```python
from build123d import *

# Parameters (mm, degrees)
BOSS_EXTRUDE1_START = -10
SKETCH2_R           = 20
BOSS_EXTRUDE1_DEPTH = 30
SKETCH5_R           = 20
SKETCH5_R_2         = 11
CUT_EXTRUDE1_DEPTH  = 10
SKETCH7_R           = 20
BOSS_EXTRUDE2_DEPTH = 50
CUT_EXTRUDE2_DEPTH  = 50
CUT_EXTRUDE3_START  = -7.5
CUT_EXTRUDE3_DEPTH  = 87.335902125
SKETCH10_R          = 7
CUT_EXTRUDE4_DEPTH  = 77.23263398


with BuildPart() as part:
    # Sketch2 → Boss-Extrude1 (new body)
    with BuildSketch(Plane.XY.offset(BOSS_EXTRUDE1_START)):
        Circle(SKETCH2_R)
    extrude(amount=BOSS_EXTRUDE1_DEPTH)

    # Sketch5 → Cut-Extrude1 (cut)
    with BuildSketch(Plane(origin=(0, 0, -10), x_dir=(-1, 0, 0), z_dir=(0, 0, -1))):
        Circle(SKETCH5_R)
        Circle(SKETCH5_R_2, mode=Mode.SUBTRACT)
    extrude(amount=-CUT_EXTRUDE1_DEPTH, mode=Mode.SUBTRACT)

    # Sketch7 → Boss-Extrude2 (add)
    with BuildSketch(Plane.XY.offset(20)):
        with Locations(Location((0, 0, 0), (0, 0, 180))):
            Circle(SKETCH7_R)
    extrude(amount=BOSS_EXTRUDE2_DEPTH)

    # Sketch8 → Cut-Extrude2 (cut)
    with BuildSketch(Plane.XY.offset(70)):
        with BuildLine():
            ThreePointArc((15, 0), (13.608051098, 6.310383928), (9.690540625, 11.449603591))
            Line((9.690540625, 11.449603591), (10.389343078, -10.819498621))
            ThreePointArc((10.389343078, -10.819498621), (13.799277991, -5.880469957), (15, 0))
        make_face()
    extrude(amount=-CUT_EXTRUDE2_DEPTH, mode=Mode.SUBTRACT)

    # Sketch9 → Cut-Extrude3 (cut, through all)
    with BuildSketch(Plane(origin=(10.039941851, 0.315052485, 0), x_dir=(0, 0, -1), z_dir=(0.9995080138957542, 0.03136447286604987, 0)).offset(CUT_EXTRUDE3_START)):
        with BuildLine():
            Line((-39.352049218, 14.5), (-72.599055299, 14.5))
            Line((-72.599055299, 14.5), (-72.599055299, -14.5))
            Line((-72.599055299, -14.5), (-39.352049218, -14.5))
            ThreePointArc((-39.352049218, -14.5), (-24.852049218, 0), (-39.352049218, 14.5))
        make_face()
    extrude(amount=CUT_EXTRUDE3_DEPTH, mode=Mode.SUBTRACT)

    # Sketch10 → Cut-Extrude4 (cut, through all)
    with BuildSketch(Plane(origin=(2.543631747, 0.079818939, 0), x_dir=(0, 0, -1), z_dir=(0.9995080138957542, 0.03136447286604988, 0))):
        with Locations(Location((-37.473518474, 0, 0), (0, 0, 90))):
            Circle(SKETCH10_R)
    extrude(amount=-CUT_EXTRUDE4_DEPTH, mode=Mode.SUBTRACT)


solid = part.part
```
For this review, take the finished solid that the model builds, in its own axes (mm). A direction names the side the tool comes from. Give positions to 0.01 mm unless a question says otherwise; leave off trailing zeros. Write each loop counter-clockwise with the first axis right and the second up, starting at its lowest first coordinate (ties: lowest second). Pieces come first, ordered by that corner, then holes.
Item 1: Take a section at C-C (z = 53). Give the boundary of the cut face in (x, y).
Item 2: The part is to be moulded in two halves that separate along X. For faces 1 (the face through (12, 0, 20)), 2 (the face through (2.38, -10.74, -5.07)), 3 (the face through (-9, -9, 0)), say which applies: +X half, -X half, draft (parallel to the pull), parting line (faces both ways), or undercut.
Item 3: Take a section at D-D (z = 9). Give the boundary of the cut face in (x, y).
Item 4: Take a section at A-A (z = 21). Give the boundary of the cut face in (x, y).
Item 5: Insertion check: P1, Ø1.5, axis at x = -7.5, z = 45, coming from the -Y side; P2, Ø2, axis at y = 5.5, z = 19.5, coming from the -X side; P3, Ø2, axis at y = 10.5, z = 1.5, coming from the +X side. Each pin has a flat end and moves straight along its axis. Give the tip position at first contact, or say it passes through.
Item 6: Take a section at B-B (y = -16). Give the boundary of the cut face in (x, z).
Item 7: Machinability: for faces 4 (the face through (-8.537, -1.18, 44.414)), 5 (the face through (9.218, -0.03, 24.856)), 6 (the face through (0, 0, -10)), which of the approach directions +Z, -Z, +X, -X, +Y, -Y give a long, thin tool a straight path to every point of the face, cutting with its end or side? Answer none if there is none.
Item 8: Wall thickness on probe 1 along Z at (x, y) = (16.5, 0.5); probe 2 along Z at (x, y) = (4.5, 0.5); probe 3 along Z at (x, y) = (-17.5, -4): over which ranges is each line inside the solid? List them lowest first.
Established:
1. outline: (2.09, 14.57) - (13.31, 14.92) arc R20 ccw (long way) to (14.22, -14.06) - (3, -14.41) - close
2. face 1: undercut
2. face 2: parting line
2. face 3: draft
3. outline: circle Ø40 at (0, 0)
4. outline: circle Ø40 at (0, 0); hole (9.69, 11.45) - (10.39, -10.82) arc R15 ccw to start
5. P1: stops at y = -18.83
5. P2: stops at x = -19.49
5. P3: stops at x = 17.6
6. outline: (-12, 0) - (12, 0) - (12, 70) - (-12, 70) - close
7. face 4: none
7. face 5: +Z
7. face 6: -Z, +X, -X, +Y, -Y
8. probe 1: z = 0 to 24.85
8. probe 2: z = -10 to 24.86
8. probe 3: z = 0 to 31.38, 43.56 to 70
